For this review, take the finished solid that the model builds, in its own axes (mm). A direction names the side the tool comes from. Give positions to 0.01 mm unless a question says otherwise; leave off trailing zeros. Write each loop counter-clockwise with the first axis right and the second up, starting at its lowest first coordinate (ties: lowest second). Pieces come first, ordered by that corner, then holes.
1) Draft analysis for pull direction Z (two halves, no side actions). For faces 4 (the face through (1, 1, 0)), 5 (the face through (1, 2, 4)), 6 (the face through (1.48, 1.76, -6.01)), state which applies: pulls with the +Z half, pulls with the -Z half, needs draft (parallel to the pull), parting line crosses it, or undercut.
2) We need section D-D on z = -4. Give the boundary of the cut face in (x, y).
3) We need section A-A on x = 2.25. Give the boundary of the cut face in (y, z).
4) Machinability: for faces 1 (the face through (1, 3, -6)), 2 (the face through (1.48, 1.74, 5.99)), 3 (the face through (1, 3, 6)), which of the approach directions +Z, -Z, +X, -X, +Y, -Y give a long, thin tool a straight path to every point of the face, cutting with its end or side? Answer none if there is none.
5) We need section B-B on z = 0. Give the boundary of the cut face in (x, y), and give its area (3 significant figures).
6) We need section C-C on y = 3.25. Give the boundary of the cut face in (x, z), and give its area (3 significant figures).
7) Wall thickness on line 1 along Y through (x, z) = (0.35, 0); line 2 along Z through (x, y) = (0.95, 2.25); line 3 along Z through (x, y) = (2.1, 3.25): over which ranges is each line inside the solid? List them lowest first.
8) For P1, Ø1, axis at x = 2, z = 1.5, coming from the +Y side; P2, Ø1, axis at x = 1.5, y = 9.5, coming from the -Z side; P3, Ø1.6, axis at x = 1.5, z = -6, coming from the +Y side, all flat-tipped, find the tip position at first contact; note any pin that passes through.
Autodesk Inventor part; units mm, degrees
ref_plane "YZ Plane" through (0, 0, 0) normal (1, 0, 0) x (0, 1, 0)
ref_plane "XZ Plane" through (0, 0, 0) normal (0, 1, 0) x (-1, 0, 0)
ref_plane "XY Plane" through (0, 0, 0) normal (0, 0, 1) x (1, 0, 0)
sketch "スケッチ1" plane through (0, 0, 0) normal (1, 0, 0) x (0, 1, 0)
  line L0 (9, 0) -> (-9, 0) construction
  line L1 (9, 3) -> (-9, 3)
  line L2 (-9, -3) -> (9, -3)
  arc A0 (9, -3) -> (9, 3) centre (9, 0) ccw
  arc A1 (-9, 3) -> (-9, -3) centre (-9, 0) ccw
  line L3 (3, 7) -> (-3, 7)
  line L4 (-3, -7) -> (3, -7)
  line L5 (3, 7) -> (-3, -7) construction
  line L6 (-3, 7) -> (3, -7) construction
  line L7 (-3, 7) -> (-3, 5)
  line L8 (3, 5) -> (3, 7)
  line L9 (3, -7) -> (3, -5)
  line L10 (3, -3) -> (3, 3)
  line L11 (-3, 3) -> (-3, -3)
  line L12 (-3, -5) -> (-3, -7)
  circle A2 centre (-9, 0) radius 1.25
  circle A3 centre (9, 0) radius 1.25
  line L13 (3, -5) -> (3, -3)
  line L14 (3, 3) -> (3, 5)
  line L15 (-3, 5) -> (-3, 3)
  line L16 (-3, -3) -> (-3, -5)
  point P0 (0, 0)
  dimension "d0" = 6
  dimension "d1" = 6
  dimension "d3" = 14
  dimension "d4" = 18
  dimension "d7" = 0
  dimension "d8" = 6
  dimension "d9" = 4
  dimension "d11" = 2.5
  dimension "d12" = 2.5
extrude "押し出し1" add sketch "スケッチ1" along normal blind 3 contours A0 L2 L10 L1 | L10 L2 L11 L1 | L1 L15 L7 L3 L8 L14 | L11 L2 A1 L1 | L13 L9 L4 L12 L16 L2 | A2 | A3
sketch "スケッチ2" plane through (0, 0, 0) normal (-1, 0, 0) x (0, 0, 1)
  circle A0 centre (0, 9) radius 1.25
  circle A1 centre (0, -9) radius 1.25
  line L0 (-3, 3) -> (-7, 3)
  line L1 (-7, 3) -> (-7, -3)
  line L2 (-7, -3) -> (-3, -3)
  line L3 (-3, -3) -> (-3, -9)
  arc A2 (-3, -9) -> (3, -9) centre (0, -9) ccw
  line L4 (3, -9) -> (3, -3)
  line L5 (3, -3) -> (7, -3)
  line L6 (7, -3) -> (7, 3)
  line L7 (7, 3) -> (3, 3)
  line L8 (3, 3) -> (3, 9)
  arc A3 (3, 9) -> (-3, 9) centre (0, 9) ccw
  line L9 (-3, 9) -> (-3, 3)
  line L10 (-7, 2.5) -> (-5, 1)
  line L11 (-5, 1) -> (5, 1)
  line L12 (5, 1) -> (7, 2.5)
  line L13 (3, 3) -> (3, 9)
  line L14 (-3, 9) -> (-3, 3)
  arc A4 (-5, 3) -> (-3, 3) centre (-4, 3) ccw
  arc A5 (3, 3) -> (5, 3) centre (4, 3) ccw
  point P0 (0, 0)
  point P1 (0, 1)
  dimension "d17" = 10
  dimension "d18" = 2
  dimension "d19" = 0.5
  dimension "d26" = 2
extrude "押し出し4" cut sketch "スケッチ2" against normal through all contours L9 A3 L8 A5 L7 L6 L12 L11 L10 L1 L0 A4 keep common part
properties part number "tip3" material "アルミニウム 2014-T4"
Results list:
1. face 4: needs draft
1. face 5: undercut
1. face 6: pulls with the -Z half
2. outline: (0, 1) - (3, 1) - (3, 2) - (0, 2) - close
3. outline: (1, -5) - (2.5, -7) - (3, -7) - (3, -5) arc R1 cw to (3, -3) - (9, -3) arc R3 ccw to (9, 3) - (3, 3) arc R1 cw to (3, 5) - (3, 7) - (2.5, 7) - (1, 5) - close; hole circle Ø2.5 at (9, 0)
4. face 1: -Z, +X, -X, +Y
4. face 2: +Z, +X, -X, -Y
4. face 3: +Z, +X, -X, +Y
5. outline: (0, 1) - (3, 1) - (3, 7.75) - (0, 7.75) - close; (0, 10.25) - (3, 10.25) - (3, 12) - (0, 12) - close
5. area: 25.5 mm2
6. outline: (0, -3) - (3, -3) - (3, 3) - (0, 3) - close
6. area: 18.0 mm2
7. line 1: y = 1 to 7.75, 10.25 to 12
7. line 2: z = -6.67 to -4.66, -3.34 to 3.34, 4.66 to 6.67
7. line 3: z = -3 to 3
8. P1: stops at y = 11.83
8. P2: stops at z = -3
8. P3: stops at y = 3
